from build123d import *

# Parameters (mm, degrees)
CUT_EXTRUDE1_DEPTH = 35
CHAMFER2_SIZE      = 1


with BuildPart() as part:
    # Sketch1 → Revolve1 (revolve)
    with BuildSketch(Plane.XY):
        with BuildLine():
            Line((0, 0), (0, 11))
            Line((0, 11), (63, 11))
            Line((63, 11), (63, 7))
            ThreePointArc((63, 7), (63.292893219, 6.292893219), (64, 6))
            Line((64, 6), (108, 6))
            Line((108, 6), (108, 0))
            Line((108, 0), (0, 0))
        make_face()
    revolve(axis=Axis((113.833823868, 0, 0), (-1, 0, 0)))

    # Sketch2 → Cut-Extrude1 (cut)
    with BuildSketch(Plane.ZY):
        with BuildLine():
            Line((-9.3, -2.5), (-6.538348415, -2.5))
            ThreePointArc((-6.538348415, -2.5), (7, 0), (-6.538348415, 2.5))
            Line((-6.538348415, 2.5), (-9.3, 2.5))
            Line((-9.3, 2.5), (-9.3, -2.5))
        make_face()
    extrude(amount=-CUT_EXTRUDE1_DEPTH, mode=Mode.SUBTRACT)

    # Chamfer2
    chamfer2_edges = [part.edges().sort_by_distance(p)[0] for p in [
        (0, 0, 7),
        (0, -11, 0),
        (63, -11, 0),
        (108, -6, 0),
    ]]
    chamfer(chamfer2_edges, length=CHAMFER2_SIZE)


solid = part.part
Work out the finished part from the listing and answer in its coordinate system (mm). A direction names the side the tool comes from. Coordinates: 2 decimals unless noted, no trailing zeros. Write each loop counter-clockwise with the first axis right and the second up, starting at its lowest first coordinate (ties: lowest second). Pieces come first, ordered by that corner, then holes. Notation, with made-up numbers: M 51,-35 L 79,-35 A28 cw 79,-16 Z; hole C -16.75,-29 d10. An arc over 180 degrees is marked long. Answer as CSV lines item,"result". Start each with the question number.
Item 1: Section C-C on x = 68 is taken. Write down the section's boundary in (y, z), and give its area (3 significant figures).
Item 2: Section B-B on x = 28 is taken. Write down the section's boundary in (y, z), and give its area (3 significant figures).
Item 3: Determine the mould class of faces 1 (the face through (17, 0, -9.3)), 2 (the face through (0, 6, 6)), 3 (the face through (86, -6, 0)) for opening direction Y: released by +Y, released by -Y, zero draft, split by the parting line, or undercut.
Item 4: Consider L1, parallel to X at y = 7.75, z = -4; L2, parallel to X at y = 0.5, z = -4.25; L3, parallel to Z at x = 43.5, y = 0. Determine where each line is inside the solid, lowest interval first.
Item 5: Flat-ended cylindrical pins translate along their axes: P1, Ø0.8, axis at x = 11, z = -8, coming from the -Y side; P2, Ø10, axis at x = 13, z = -5, coming from the +Y side; P3, Ø2, axis at x = 68, y = -3.5, coming from the +Z side; P4, Ø8, axis at x = 71, z = -6, coming from the -Y side. Find the tip coordinate at first contact, or state that the pin passes through.
Item 6: Section D-D on x = 49 is taken. Write down the section's boundary in (y, z), and give its area (3 significant figures).
Item 7: A tool of negligible diameter and unlimited length cuts with its end or side. For faces 4 (the face through (17, -2.5, -8)), 5 (the face through (31.93, -2.38, 10.74)), 6 (the face through (63, 2, -7)), from which of +Z, -Z, +X, -X, +Y, -Y can it reach the whole face along a straight path? Write none if from no direction.
Item 8: Section A-A on y = 0 is taken. Write down the section's boundary in (x, z).
Checks:
1,outline,"C 0,0 d12"
1,area,"113 mm²"
2,outline,"C 0,0 d22; hole M -2.5,-9.3 L 2.5,-9.3 L 2.5,-6.54 A7 ccw long -2.5,-6.54 Z"
2,area,"214 mm²"
3,face 1,"undercut"
3,face 2,"zero draft"
3,face 3,"split by the parting line"
4,L1,"x = 0 to 63"
4,L2,"x = 35 to 108"
4,L3,"z = -11 to 11"
5,P1,"stops at y = -7.95"
5,P2,"stops at y = 11"
5,P3,"stops at z = 5.45"
5,P4,"stops at y = -5.66"
6,outline,"C 0,0 d22"
6,area,"380 mm²"
7,face 4,"-X"
7,face 5,"+X, -X"
7,face 6,"+X"
8,outline,"M 0,-10 L 1,-11 L 62,-11 L 63,-10 L 63,-7 A1 cw 64,-6 L 107,-6 L 108,-5 L 108,5 L 107,6 L 64,6 A1 cw 63,7 L 63,10 L 62,11 L 1,11 L 0,10 L 0,8 L 1,7 L 35,7 L 35,-9.3 L 0,-9.3 Z"
